```python
from build123d import *

# Parameters (mm, degrees)
SALIENTE_EXTRUIR1_DEPTH = 3.1242
CROQUIS2_R              = 1.651
CORTAR_EXTRUIR1_DEPTH   = 4.1242
CROQUIS3_R              = 1.651
CORTAR_EXTRUIR2_DEPTH   = 3.1242
CROQUIS4_R              = 14.1097
CROQUIS4_R_2            = 1.5367
CORTAR_EXTRUIR3_DEPTH   = 4.1242


with BuildPart() as part:
    # Croquis1 → Saliente-Extruir1 (new body)
    with BuildSketch(Plane.XY):
        with BuildLine():
            Line((-53.975, -47.625), (53.975, -47.625))
            ThreePointArc((53.975, -47.625), (60.710192091, -44.835192091), (63.5, -38.1))
            Line((63.5, -38.1), (63.5, 38.1))
            ThreePointArc((63.5, 38.1), (60.710192091, 44.835192091), (53.975, 47.625))
            Line((53.975, 47.625), (-53.975, 47.625))
            ThreePointArc((-53.975, 47.625), (-60.710192091, 44.835192091), (-63.5, 38.1))
            Line((-63.5, 38.1), (-63.5, -38.1))
            ThreePointArc((-63.5, -38.1), (-60.710192091, -44.835192091), (-53.975, -47.625))
        make_face()
    extrude(amount=SALIENTE_EXTRUIR1_DEPTH)

    # Croquis2 → Cortar-Extruir1 (cut, through all)
    with BuildSketch(Plane.XY.offset(3.1242)):
        with Locations((-41.275, 44.45)):
            Circle(CROQUIS2_R)
        with Locations((41.275, 44.45)):
            Circle(CROQUIS2_R)
        with Locations((41.275, -44.45)):
            Circle(CROQUIS2_R)
        with Locations((-41.275, -44.45)):
            Circle(CROQUIS2_R)
    extrude(amount=-CORTAR_EXTRUIR1_DEPTH, mode=Mode.SUBTRACT)

    # Croquis3 → Cortar-Extruir2 (cut)
    with BuildSketch(Plane(origin=(0, 0, 0), x_dir=(-1, 0, 0), z_dir=(0, 0, -1))):
        with BuildLine():
            ThreePointArc((-27.5625, 12.225), (-44.886616139, 5.049116139), (-52.0625, -12.275))
            Line((-52.0625, -12.275), (-27.5625, -12.275))
            Line((-27.5625, -12.275), (-27.5625, 12.225))
        make_face()
        with BuildLine():
            Line((-27.5625, -12.275), (-52.0625, -12.275))
            ThreePointArc((-52.0625, -12.275), (-44.886616139, -29.599116139), (-27.5625, -36.775))
            Line((-27.5625, -36.775), (-27.5625, -12.275))
        make_face()
        with BuildLine():
            Line((-27.5625, 12.225), (-27.5625, -12.275))
            Line((-27.5625, -12.275), (-3.0625, -12.275))
            ThreePointArc((-3.0625, -12.275), (-10.238383861, 5.049116139), (-27.5625, 12.225))
        make_face()
        with BuildLine():
            Line((-3.0625, -12.275), (-27.5625, -12.275))
            Line((-27.5625, -12.275), (-27.5625, -36.775))
            ThreePointArc((-27.5625, -36.775), (-10.238383861, -29.599116139), (-3.0625, -12.275))
        make_face()
        with Locations((-3.0625, 16.725)):
            Circle(CROQUIS3_R)
        with Locations((-52.0625, 16.725)):
            Circle(CROQUIS3_R)
        with Locations((-52.0625, -41.275)):
            Circle(CROQUIS3_R)
        with Locations((-3.0625, -41.275)):
            Circle(CROQUIS3_R)
    extrude(amount=-CORTAR_EXTRUIR2_DEPTH, mode=Mode.SUBTRACT)

    # Croquis4 → Cortar-Extruir3 (cut, through all)
    with BuildSketch(Plane(origin=(0, 0, 0), x_dir=(-1, 0, 0), z_dir=(0, 0, -1))):
        with Locations((36.6903, 9.8552)):
            Circle(CROQUIS4_R)
        with Locations((35.7378, 31.75)):
            Circle(CROQUIS4_R_2)
        with Locations((50.8, 31.75)):
            Circle(CROQUIS4_R_2)
        with Locations((50.8, -12.0396)):
            Circle(CROQUIS4_R_2)
        with Locations((22.5806, -12.0396)):
            Circle(CROQUIS4_R_2)
        with BuildLine():
            Line((11.1633, -26.2763), (49.2633, -26.2763))
            ThreePointArc((49.2633, -26.2763), (55.6133, -32.6263), (49.2633, -38.9763))
            Line((49.2633, -38.9763), (11.1633, -38.9763))
            ThreePointArc((11.1633, -38.9763), (4.8133, -32.6263), (11.1633, -26.2763))
        make_face()
    extrude(amount=-CORTAR_EXTRUIR3_DEPTH, mode=Mode.SUBTRACT)


solid = part.part
```
For this review, take the finished solid that the model builds, in its own axes (mm). A direction names the side the tool comes from. Round coordinates to 2 decimals unless told otherwise and drop trailing zeros. Order: outer loops, then holes, each group sorted by start corner. A loop starts at its lowest first (then second) coordinate and runs counter-clockwise, first axis right, second up. Notation, with made-up numbers: (66.25, 89.25) -> (86.25, 89.25) arc R21 cw to (86.25, 117.25) -> close; hole circle Ø3 at (-24.75, 15). An arc over 180 degrees is marked (long way). Use a Markdown table: item, result.
Item 1: For line 1 along Y through (x, z) = (-11.5, 1.85) (3 decimals); line 2 along Y through (x, z) = (-25, 0.4) (3 decimals); line 3 along X through (y, z) = (-28, 0.85), list the stretches that pass through material, from the lowest coordinate up. Write a range as [from, to].
Resolved:
| item | result |
|---|---|
| line 1 | y = [-47.625, -38.976], [-26.276, 47.625] |
| line 2 | y = [-47.625, -38.976], [-26.276, 1.955], [17.756, 47.625] |
| line 3 | x = [-63.5, -53.61], [-6.81, 8.77], [46.35, 63.5] |
Item 2: Take a section at B-B (x = 37.5). State the section outline as (y, z) points (3 decimals), plus the area to 3 significant figures.
Resolved:
| item | result |
|---|---|
| outline | (-47.625, 0) -> (-34.669, 0) -> (-34.669, 3.124) -> (-47.625, 3.124) -> close; (10.119, 0) -> (47.625, 0) -> (47.625, 3.124) -> (10.119, 3.124) -> close |
| area | 158 mm² |
Item 3: Draft analysis for pull direction X (two halves, no side actions). For faces 3 (the cylindrical face through (53.28, 17.84, 1.54)), 4 (the flat face through (-63.5, 1, 2)), 5 (the cylindrical face through (42.8, -45.08, 1.58)), 6 (the flat face through (-1, 1, 3.124)), state which applies: +X half, -X half, draft (parallel to the pull), parting line (faces both ways), or undercut.
Resolved:
| item | result |
|---|---|
| face 3 | undercut |
| face 4 | -X half |
| face 5 | undercut |
| face 6 | draft |
Item 4: Take a section at C-C (z = 2.05). State how many separate pieces and enclosed holes the cut face has, plus the area to 3 significant figures.
Resolved:
| item | result |
|---|---|
| separate pieces | 1 |
| enclosed holes | 15 |
| area | 8,800 mm² |
Item 5: Take a section at A-A (y = 31.75). State the section outline as (x, z) points.
Resolved:
| item | result |
|---|---|
| outline | (-63.5, 0) -> (-52.34, 0) -> (-52.34, 3.12) -> (-63.5, 3.12) -> close; (-49.26, 0) -> (-37.27, 0) -> (-37.27, 3.12) -> (-49.26, 3.12) -> close; (-34.2, 0) -> (63.5, 0) -> (63.5, 3.12) -> (-34.2, 3.12) -> close |
Item 6: For pin 1 (2.5 mm diameter, centred on x = -50.8, y = -12.04, fed in from +Z), flat-tipped, find the tip position at first contact; note if it passes through.
Resolved:
| item | result |
|---|---|
| pin 1 | passes through |
Item 7: Take a section at D-D (y = 6.5). State the section outline as (x, z) points.
Resolved:
| item | result |
|---|---|
| outline | (-63.5, 0) -> (-50.4, 0) -> (-50.4, 3.12) -> (-63.5, 3.12) -> close; (-22.99, 0) -> (11.82, 0) -> (11.82, 3.12) -> (-22.99, 3.12) -> close; (43.3, 0) -> (63.5, 0) -> (63.5, 3.12) -> (43.3, 3.12) -> close |
Item 8: Machinability: for faces 1 (the cylindrical face through (-4.815, -32.766, 1.54)), 2 (the cylindrical face through (-60.784, -44.761, 1.54)), which of the approach directions +Z, -Z, +X, -X, +Y, -Y give a long, thin tool a straight path to every point of the face, cutting with its end or side? Answer none if there is none.
Resolved:
| item | result |
|---|---|
| face 1 | +Z, -Z |
| face 2 | +Z, -Z, -X, -Y |
